Here's how the part is built. I have some questions about the finished solid (model axes, mm). Face numbers are marked on the shaded views. A direction names the side the tool comes from. Round coordinates to 2 decimals unless told otherwise and drop trailing zeros. Write each loop counter-clockwise with the first axis right and the second up, starting at its lowest first coordinate (ties: lowest second). Pieces come first, ordered by that corner, then holes. Notation, with made-up numbers: M 63.5,-5.75 L 69.5,-5.75 A32 ccw 69.5,28.25 Z; hole C -8,-16.5 d4. An arc over 180 degrees is marked long. Write item = value, one per line. Start each with the question number.
(1) I want a section at A-A (y = 0). List the corners of the cut face in (x, z) for me, and give its area (3 significant figures).
(2) Will these pins go through, and if not, where does the flat tip stop? pin 1 Ø1.5 at (x, y) = (3, -3.5) entering from +Z; pin 2 Ø4 at (x, y) = (9, 4) entering from -Z; pin 3 Ø3 at (x, z) = (7.5, 39.5) entering from -Y; pin 4 Ø1.2 at (y, z) = (9.5, -2) entering from -X.
(3) I want a section at D-D (x = -10). List the corners of the cut face in (y, z) for me, and give its area (3 significant figures).
(4) I want a section at B-B (z = 10.5). List the corners of the cut face in (x, y) for me.
(5) I want a section at C-C (y = 9.5). List the corners of the cut face in (x, z) for me, and give its area (3 significant figures).
(6) On a 3-axis mill with a long thin cutter (end or side, diameter ignored), from which of +Z, -Z, +X, -X, +Y, -Y can I reach the whole of each face in a straight line? I mean the marked faces 1 and 2. Say none if no direction works.
(7) I need wall thicknesses on line 1 along Y through (x, z) = (-0.15, -2); line 2 along Z through (x, y) = (0, -9.5); line 3 along Z through (x, y) = (1.25, 11.25). Which ranges of each line are inside material? Lowest first, please.
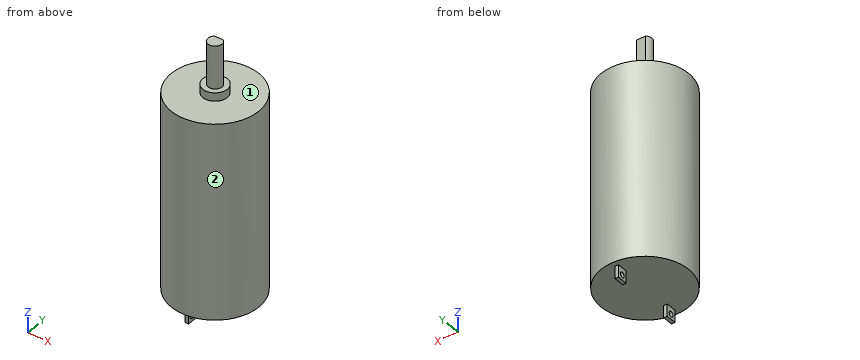
```python
from build123d import *

# Parameters (mm, degrees)
SKETCH1_R               = 12.5
BOSS_EXTRUDE1_DEPTH     = 55.8
BOSS_EXTRUDE2_START     = 55.8
SKETCH2_R               = 3.5
BOSS_EXTRUDE2_DEPTH     = 2.38
BOSS_EXTRUDE3_START     = 58.18
SKETCH3_R               = 2
BOSS_EXTRUDE3_DEPTH     = 12.2
SKETCH5_W               = 2.645751312
SKETCH5_H               = 1.197132969
CUT_EXTRUDE1_DEPTH      = 12.2
SKETCH6_W               = 1
SKETCH6_H               = 3
BOSS_EXTRUDE4_DEPTH     = 3.5
CUT_EXTRUDE2_DEPTH      = 73.566138109
CUT_EXTRUDE2_DEPTH_BACK = 73.566138109
SKETCH7_R               = 0.75


with BuildPart() as part:
    # Sketch1 → Boss-Extrude1 (new body)
    with BuildSketch(Plane.XY):
        Circle(SKETCH1_R)
    extrude(amount=BOSS_EXTRUDE1_DEPTH)

    # Sketch2 → Boss-Extrude2 (add)
    with BuildSketch(Plane.XY.offset(BOSS_EXTRUDE2_START)):
        Circle(SKETCH2_R)
    extrude(amount=BOSS_EXTRUDE2_DEPTH)

    # Sketch3 → Boss-Extrude3 (add)
    with BuildSketch(Plane.XY.offset(BOSS_EXTRUDE3_START)):
        Circle(SKETCH3_R)
    extrude(amount=BOSS_EXTRUDE3_DEPTH)

    # Sketch5 → Cut-Extrude1 (cut)
    with BuildSketch(Plane.XY.offset(58.18)):
        with Locations((0, 2.098566485)):
            Rectangle(SKETCH5_W, SKETCH5_H)
    extrude(amount=CUT_EXTRUDE1_DEPTH, mode=Mode.SUBTRACT)

    # Sketch6 → Boss-Extrude4 (add)
    with BuildSketch(Plane.XY):
        with Locations((0, 9.5)):
            Rectangle(SKETCH6_W, SKETCH6_H)
        with Locations((0, -9.5)):
            Rectangle(SKETCH6_W, SKETCH6_H)
    extrude(amount=-BOSS_EXTRUDE4_DEPTH)

    # Sketch7 → Cut-Extrude2 (cut, two sides: drawn at the far end of the back side and taken through both)
    with BuildSketch(Plane(origin=(0, 0, 0), x_dir=(0, 0, -1), z_dir=(1, 0, 0)).offset(-CUT_EXTRUDE2_DEPTH_BACK)):
        with Locations(Location((2, 9.5, 0), (0, 0, 90))):
            Circle(SKETCH7_R)
        with Locations(Location((2, -9.5, 0), (0, 0, 90))):
            Circle(SKETCH7_R)
    extrude(amount=CUT_EXTRUDE2_DEPTH + CUT_EXTRUDE2_DEPTH_BACK, mode=Mode.SUBTRACT)


solid = part.part
```
Returned:
q1.outline = M -12.5,0 L 12.5,0 L 12.5,55.8 L 3.5,55.8 L 3.5,58.18 L 2,58.18 L 2,70.38 L -2,70.38 L -2,58.18 L -3.5,58.18 L -3.5,55.8 L -12.5,55.8 Z
q1.area = 1,460 mm²
q2.pin_1 = 55.8
q2.pin_2 = 0
q2.pin_3 = -10.97
q2.pin_4 = through
q3.outline = M -7.5,0 L 7.5,0 L 7.5,55.8 L -7.5,55.8 Z
q3.area = 837 mm²
q4.outline = C 0,0 d25
q5.outline = M -8.12,0 L -0.5,0 L -0.5,-1.25 L 0.5,-1.25 L 0.5,0 L 8.12,0 L 8.12,55.8 L -8.12,55.8 Z; M -0.5,-3.5 L 0.5,-3.5 L 0.5,-2.75 L -0.5,-2.75 Z
q5.area = 909 mm²
q6.face_1 = +Z
q6.face_2 = +Z, -Z
q7.line_1 = -11 to -10.25, -8.75 to -8, 8 to 8.75, 10.25 to 11
q7.line_2 = -3.5 to -2.75, -1.25 to 55.8
q7.line_3 = 0 to 55.8
